```python
from build123d import *

# Parameters (mm, degrees)
BOSS_EXTRUDE1_DEPTH          = 32.251106428
SKETCH2_W                    = 29.251106428
SKETCH2_H                    = 41.502212856
CUT_EXTRUDE1_DEPTH           = 107.913538909
SKETCH3_W                    = 29.251106428
SKETCH3_H                    = 79.251106428
CUT_EXTRUDE2_DEPTH           = 107.913538909
SKETCH4_W                    = 8
SKETCH4_H                    = 2.5
CUT_EXTRUDE3_DEPTH           = 116.523199892
F_3_0_3_DIAMETER_HOLE1_D     = 3
F_3_0_3_DIAMETER_HOLE1_DEPTH = 32.251106428
FILLET1_R                    = 2
FILLET2_R                    = 5


with BuildPart() as part:
    # Sketch1 → Boss-Extrude1 (new body)
    with BuildSketch(Plane(origin=(-23.875925357, 0, 0), x_dir=(0, 0, -1), z_dir=(1, 0, 0))):
        with BuildLine():
            Line((-65.19367103, 82.251106428), (-65.19367103, -41.502212856))
            Line((-65.19367103, -41.502212856), (-50.19367103, -41.502212856))
            Line((-50.19367103, -41.502212856), (-50.19367103, 82.251106428))
            ThreePointArc((-50.19367103, 82.251106428), (-57.69367103, 89.751106428), (-65.19367103, 82.251106428))
        make_face()
    extrude(amount=-BOSS_EXTRUDE1_DEPTH)

    # Sketch2 → Cut-Extrude1 (cut, through all)
    with BuildSketch(Plane.XY.offset(65.19367103)):
        with Locations((-38.501478571, -20.751106428)):
            Rectangle(SKETCH2_W, SKETCH2_H)
    extrude(amount=-CUT_EXTRUDE1_DEPTH, mode=Mode.SUBTRACT)

    # Sketch3 → Cut-Extrude2 (cut, through all)
    with BuildSketch(Plane.XY.offset(65.19367103)):
        with Locations((-41.501478571, 50.125553214)):
            Rectangle(SKETCH3_W, SKETCH3_H)
    extrude(amount=-CUT_EXTRUDE2_DEPTH, mode=Mode.SUBTRACT)

    # Sketch4 → Cut-Extrude3 (cut, through all)
    with BuildSketch(Plane.ZY.offset(56.127031785)):
        with Locations((59.19367103, -40.252212856)):
            Rectangle(SKETCH4_W, SKETCH4_H)
    extrude(amount=-CUT_EXTRUDE3_DEPTH, mode=Mode.SUBTRACT)

    # Ø3.0 (3) Diameter Hole1
    with Locations(Plane(origin=(-23.875925357, 0, 0), x_dir=(0, 0, -1), z_dir=(1, 0, 0))):
        with Locations((-57.69367103, 67.251106428)):
            Hole(F_3_0_3_DIAMETER_HOLE1_D / 2, depth=F_3_0_3_DIAMETER_HOLE1_DEPTH)

    # Fillet1
    fillet1_edges = [part.edges().sort_by_distance(p)[0] for p in [
        (-53.127031785, 0, 57.69367103),
        (-26.875925357, 10.5, 57.69367103),
    ]]
    fillet(fillet1_edges, radius=FILLET1_R)

    # Fillet2
    fillet2_edges = [part.edges().sort_by_distance(p)[0] for p in [
        (-23.875925357, 0, 57.69367103),
        (-56.127031785, 10.5, 57.69367103),
    ]]
    fillet(fillet2_edges, radius=FILLET2_R)


solid = part.part
```
Verification items for the finished model (mm, model axes). A direction names the side the tool comes from. Give positions to 0.01 mm unless a question says otherwise; leave off trailing zeros. Order: outer loops, then holes, each group sorted by start corner. A loop starts at its lowest first (then second) coordinate and runs counter-clockwise, first axis right, second up. Notation, with made-up numbers: (35.25, -30.75) - (92.25, -30.75) arc R21 ccw to (92.25, 5.25) - close; hole circle Ø3 at (11, 16.5). An arc over 180 degrees is marked (long way). Answer as CSV lines item,"result". Start each with the question number.
Item 1: Access from +Z, -Z, +X, -X, +Y, -Y to the whole of each face (thin tool, end or side, straight path). Record for faces 4 (the face through (-55, -40, 63.194)), 5 (the face through (-40, 0, 58)), 6 (the face through (-40, 10.5, 58)).
Item 2: Section check D-D, the plane x = -25.5. Record the boundary of the cut face in (y, z), plus the area to 3 significant figures.
Item 3: Mould release check, pull along Z, two halves, no side actions. Record for faces 1 (the face through (-36, 6, 50.194)), 2 (the face through (-23.876, 48, 58)), 3 (the face through (-55, -40, 55.194)): released by +Z, released by -Z, zero draft, split by the parting line, or undercut.
Item 4: Section check C-C, the plane x = -40. Record the boundary of the cut face in (y, z), plus the area to 4 significant figures.
Item 5: Section check A-A, the plane z = 51.75. Record the boundary of the cut face in (x, y).
Item 6: Section check B-B, the plane y = -29. Record the boundary of the cut face in (x, z).
Item 7: Gauge pin test, flat ends, axial feed: pin 1 (3 mm diameter, centred on x = -27.5, y = -2, fed in from +Z); pin 2 (4.5 mm diameter, centred on y = 41, z = 54.5, fed in from -X); pin 3 (8 mm diameter, centred on x = -46.5, z = 53, fed in from +Y); pin 4 (1 mm diameter, centred on x = -48.5, z = 54.5, fed in from -Y). Record the tip position at first contact, or that the pin passes through.
Item 8: Material ranges on L1, parallel to X at y = 53, z = 59.25; L2, parallel to X at y = -34.5, z = 58.5; L3, parallel to Y at x = -31, z = 62.75, recorded low to high.
Filled in:
1,face 4,"+X, -X, -Y"
1,face 5,"+Z, -Z, +X, -Y"
1,face 6,"+Z, -Z, -X, +Y"
2,outline,"(1.31, 50.19) - (82.25, 50.19) arc R7.5 ccw to (82.25, 65.19) - (1.31, 65.19) - close; hole circle Ø3 at (67.25, 57.69)"
2,area,"1,300 mm^2"
3,face 1,"released by -Z"
3,face 2,"zero draft"
3,face 3,"undercut"
4,outline,"(0, 50.19) - (10.5, 50.19) - (10.5, 65.19) - (0, 65.19) - close"
4,area,"157.5 mm^2"
5,outline,"(-56.13, -41.5) - (-53.13, -41.5) - (-53.13, -2) arc R2 cw to (-51.13, 0) - (-28.88, 0) arc R5 ccw to (-23.88, 5) - (-23.88, 86.83) - (-26.88, 86.83) - (-26.88, 12.5) arc R2 cw to (-28.88, 10.5) - (-51.13, 10.5) arc R5 ccw to (-56.13, 5.5) - close"
6,outline,"(-56.13, 50.19) - (-53.13, 50.19) - (-53.13, 65.19) - (-56.13, 65.19) - close"
7,pin 1,"through"
7,pin 2,"x = -26.88"
7,pin 3,"y = 10.5"
7,pin 4,"y = 0"
8,L1,"-26.88 to -23.88"
8,L2,"-56.13 to -53.13"
8,L3,"0 to 10.5"
